Model file for the job. Use its own axes, mm. Round coordinates to 2 decimals unless told otherwise and drop trailing zeros. Order: outer loops, then holes, each group sorted by start corner. A loop starts at its lowest first (then second) coordinate and runs counter-clockwise, first axis right, second up. Notation, with made-up numbers: (24, 33) -> (80, 33) arc R8 cw to (80, 46) -> close; hole circle Ø10 at (70.25, -16). An arc over 180 degrees is marked (long way). Put each result on its own line as item: value. Start each with the question number.
Q1. Cut at A-A, the plane x = -90. List the corners of the cut face in (y, z).
Q2. Probe L1, parallel to Y at x = -46, z = -28.5; L2, parallel to Y at x = -62.5, z = -10. List the from-to ranges inside material, lowest first.
Q3. Flat gauge pins, fed straight in: P1, Ø1, axis at x = -171, z = -13, coming from the +Y side; P2, Ø8, axis at x = -23, z = -4, coming from the -Y side; P3, Ø4, axis at x = -78.5, z = -4.5, coming from the +Y side; P4, Ø1, axis at x = -61.5, z = -26.5, coming from the -Y side. Where does each tip first touch, or does it go through?
Q4. Cut at B-B, the plane z = -3.5. List the corners of the cut face in (x, y), and give its area (3 significant figures).
from build123d import *

# Parameters (mm, degrees)
SALIENTE_EXTRUIR1_DEPTH                              = 200
REFRENTADO_PARA_TORNILLO_TAP_N_CON_CABEZ_D           = 3.4
REFRENTADO_PARA_TORNILLO_TAP_N_CON_CABEZ_CSINK_D     = 6.72
REFRENTADO_PARA_TORNILLO_TAP_N_CON_CABEZ_CSINK_ANGLE = 90


with BuildPart() as part:
    # Croquis1 → Saliente-Extruir1 (new body)
    with BuildSketch(Plane(origin=(0, 0, 0), x_dir=(0, 0, -1), z_dir=(1, 0, 0))):
        Polygon((0, 0), (30.909626441, 8.282209443), (31.284914057, 6.881616995), (5.602369792, 0), align=None)
    extrude(amount=-SALIENTE_EXTRUIR1_DEPTH)

    # Refrentado para tornillo tapón con cabeza plana de clavija de M31 (through all)
    with Locations(Plane(origin=(0, 0, 0), x_dir=(1, 0, 0), z_dir=(0, 0.9659258262890681, 0.2588190451025215))):
        with Locations((-190, 18), (-130, 18), (-70, 18), (-10, 18)):
            CounterSinkHole(REFRENTADO_PARA_TORNILLO_TAP_N_CON_CABEZ_D / 2, REFRENTADO_PARA_TORNILLO_TAP_N_CON_CABEZ_CSINK_D / 2, counter_sink_angle=REFRENTADO_PARA_TORNILLO_TAP_N_CON_CABEZ_CSINK_ANGLE)


solid = part.part
Ans:
1. outline: (0, -5.6) -> (6.88, -31.28) -> (8.28, -30.91) -> (0, 0) -> close
2. L1: y = 6.14 to 7.64
2. L2: y = 1.18 to 2.68
3. P1: stops at y = 3.62
3. P2: stops at y = 0
3. P3: stops at y = 1.74
3. P4: stops at y = 5.47
4. outline: (-200, 0) -> (0, 0) -> (0, 0.94) -> (-200, 0.94) -> close
4. area: 188 mm^2
